from build123d import *

# Parameters (mm, degrees)
SKETCH1_R           = 1.85
BOSS_EXTRUDE2_DEPTH = 10
FILLET2_R           = 0.3


with BuildPart() as part:
    # Sketch1 → Boss-Extrude2 (new body)
    with BuildSketch(Plane.XY):
        with BuildLine():
            ThreePointArc((1.575502084, 3.479267682), (0, 3.273519226), (-1.575502084, 3.479267682))
            ThreePointArc((-1.575502084, 3.479267682), (-5.542201702, -1.924839942), (1.04, -0.654522727))
            ThreePointArc((1.04, -0.654522727), (2.5, 1.6), (3.96, -0.654522727))
            ThreePointArc((3.96, -0.654522727), (3.740219574, -1.794341014), (3.320993506, -2.876809797))
            ThreePointArc((3.320993506, -2.876809797), (3.544154136, -3.154894829), (3.850693731, -3.337008607))
            ThreePointArc((3.850693731, -3.337008607), (5.914793747, 1.139817384), (1.575502084, 3.479267682))
        make_face()
        with Locations((-2.5, 0)):
            Circle(SKETCH1_R, mode=Mode.SUBTRACT)
    extrude(amount=BOSS_EXTRUDE2_DEPTH)

    # Fillet2
    fillet2_edges = [part.edges().sort_by_distance(p)[0] for p in [
        (1.04, -0.654522727, 5),
        (3.850693731, -3.337008607, 5),
        (3.320993506, -2.876809797, 5),
    ]]
    fillet(fillet2_edges, radius=FILLET2_R)


solid = part.part
Source: CAD feature listing. Evaluate the final solid. Frame: model axes, mm. A direction names the side the tool comes from. Round coordinates to 2 decimals unless told otherwise and drop trailing zeros. Loops run counter-clockwise (first coordinate to the right, second up) from the corner with the lowest first, then second, coordinate; pieces in that order, holes last. Notation, with made-up numbers: (81.25, 1.5) -> (123.25, 1.5) arc R36 ccw to (123.25, 36.5) -> close; hole circle Ø11 at (86, -13.5). An arc over 180 degrees is marked (long way). Answer as a JSON object with one key per item and string values. Group by question number.
Q1. Access query for faces 4 (the cylindrical face through (3.767, -1.699, 4.93)), 5 (the flat face through (0, 0, 0)). Directions: +Z, -Z, +X, -X, +Y, -Y. A direction counts if a zero-diameter tool reaches every point of the face in a straight line with its end or side. Return the directions, or none.
Q2. Ray query, line 1 (X direction, y = -1.25, z = 4); line 2 (X direction, y = -1, z = 6.75); line 3 (X direction, y = -3, z = 6.25). Return the intervals inside material, ascending. Write a range as from..to.
Q3. Mould query, pull axis Y, two halves, no side actions, for faces 1 (the cylindrical face through (0.022, 3.274, 4.93)), 2 (the cylindrical face through (-0.79, -0.71, 4.93)), 3 (the flat face through (0, 0, 10)). Classes: pulls with the +Y half, pulls with the -Y half, needs draft (parallel to the pull), parting line crosses it, or undercut.
Q4. Section query B-B (x = -2.5). Output: boundary loops of the cut face in (y, z).
Q5. Section query D-D (x = 0). Output: boundary loops of the cut face in (y, z), plus the area to 3 significant figures.
Q6. Section query C-C (y = -1). Output: boundary loops of the cut face in (x, z), plus the area to 3 significant figures.
Q7. Section query A-A (y = 0). Output: boundary loops of the cut face in (x, z), plus the area to 3 significant figures.
Q8. Contact query for flat-ended pins moving along their axis: P1, Ø3.5, axis at x = -2.5, y = 0, coming from the -Z side; P2, Ø1.5, axis at x = 3, z = 8.5, coming from the -Y side; P3, Ø3, axis at x = 2, z = 6.5, coming from the -Y side. Output: stop coordinate, or through.
Completed:
{
 "1": {"face 4": "+Z, -Z", "face 5": "-Z, +X, -X, +Y, -Y"},
 "2": {"line 1": "-5.88..-3.86, -1.14..0.88, 3.87..5.88", "line 2": "-5.96..-4.06, -0.94..0.96, 3.92..5.96", "line 3": "-4.49..-0.51, 3.4..4.49"},
 "3": {"face 1": "pulls with the +Y half", "face 2": "undercut", "face 3": "needs draft"},
 "4": {"outline": "(-3.6, 0) -> (-1.85, 0) -> (-1.85, 10) -> (-3.6, 10) -> close; (1.85, 0) -> (3.6, 0) -> (3.6, 10) -> (1.85, 10) -> close"},
 "5": {"outline": "(-2.59, 0) -> (3.27, 0) -> (3.27, 10) -> (-2.59, 10) -> close", "area": "58.6 mm²"},
 "6": {"outline": "(-5.96, 0) -> (-4.06, 0) -> (-4.06, 10) -> (-5.96, 10) -> close; (-0.94, 0) -> (0.96, 0) -> (0.96, 10) -> (-0.94, 10) -> close; (3.92, 0) -> (5.96, 0) -> (5.96, 10) -> (3.92, 10) -> close", "area": "58.5 mm²"},
 "7": {"outline": "(-6.1, 0) -> (-4.35, 0) -> (-4.35, 10) -> (-6.1, 10) -> close; (-0.65, 0) -> (0.9, 0) -> (0.9, 10) -> (-0.65, 10) -> close; (4.1, 0) -> (6.1, 0) -> (6.1, 10) -> (4.1, 10) -> close", "area": "53.0 mm²"},
 "8": {"P1": "through", "P2": "y = -3.29", "P3": "y = -3.11"}
}
